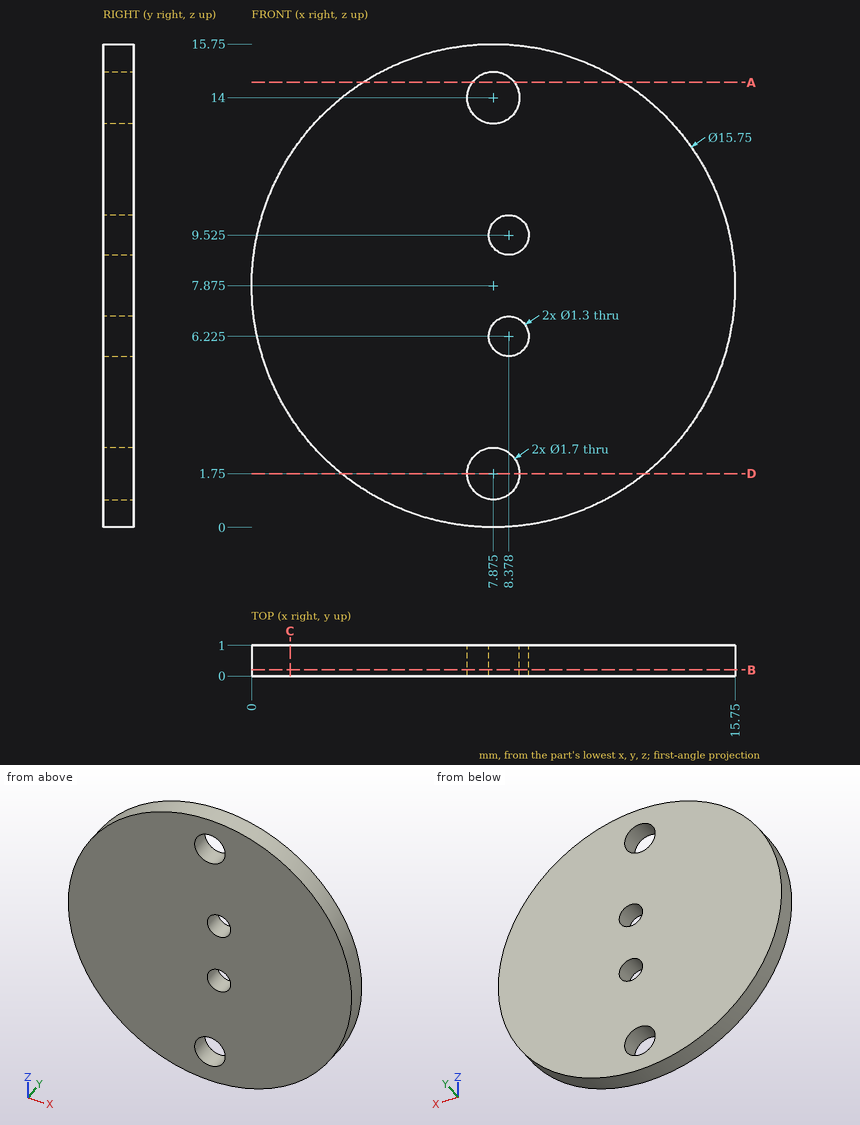
Drawing for the job (mm, zero at the part's lowest x, y, z). Coordinates: 2 decimals unless noted, no trailing zeros. Order: outer loops, then holes, each group sorted by start corner. A loop starts at its lowest first (then second) coordinate and runs counter-clockwise, first axis right, second up. Notation, with made-up numbers: (25, 43.25) - (57, 43.25) arc R32 cw to (57, 79.25) - close; hole circle Ø5 at (65.5, 82.25). An arc over 180 degrees is marked (long way). Use a Markdown table: item, result. Add a question column.
(1) Saw through at B-B (y = 0.2). Give the cut face in (x, z) (3 decimals), then the cut area to 3 significant figures.
(2) Saw through at D-D (z = 1.75). Give the cut face in (x, y) (3 decimals).
(3) Drill centre lines: line 1 along Z through (x, y) = (8.5, 0.3) (1 decimal); line 2 along X through (y, z) = (0.4, 8); line 3 along X through (y, z) = (0.35, 10) (1 decimal). Where is each one in solid material? Low to high. Write a range as [from, to].
(4) Flat gauge pin, fed straight in: pin 1 (1.4 mm diameter, centred on x = 7.875, z = 1.75, fed in from -Y). Where does the tip first touch, or does it go through?
(5) Saw through at C-C (x = 1.25). Give the cut face in (y, z).
(6) Saw through at A-A (z = 14.5). Give the cut face in (x, y), then the cut area to 3 significant figures.
Solved:
| question | item | result |
|---|---|---|
| 1 | outline | circle Ø15.75 at (7.875, 7.875); hole circle Ø1.7 at (7.875, 1.75); hole circle Ø1.7 at (7.875, 14); hole circle Ø1.3 at (8.378, 6.225); hole circle Ø1.3 at (8.378, 9.525) |
| 1 | area | 188 mm² |
| 2 | outline | (2.925, 0) - (7.025, 0) - (7.025, 1) - (2.925, 1) - close; (8.725, 0) - (12.825, 0) - (12.825, 1) - (8.725, 1) - close |
| 3 | line 1 | z = [0, 1.2], [2.3, 5.6], [6.9, 8.9], [10.2, 13.4], [14.6, 15.7] |
| 3 | line 2 | x = [0, 15.75] |
| 3 | line 3 | x = [0.3, 7.9], [8.8, 15.5] |
| 4 | pin 1 | passes through |
| 5 | outline | (0, 3.62) - (1, 3.62) - (1, 12.13) - (0, 12.13) - close |
| 6 | outline | (3.62, 0) - (7.19, 0) - (7.19, 1) - (3.62, 1) - close; (8.56, 0) - (12.13, 0) - (12.13, 1) - (8.56, 1) - close |
| 6 | area | 7.14 mm² |
